Design review of the part shown in the three views and the two pictorial views. Dimensions are in mm from the part's minimum x, y and z. Round coordinates to 2 decimals unless told otherwise and drop trailing zeros. Loops run counter-clockwise (first coordinate to the right, second up) from the corner with the lowest first, then second, coordinate; pieces in that order, holes last.
1. Consider section A-A on x = 22.5. State the section outline as (y, z) points, then the cut area to 3 significant figures.
2. Clearance check with a flat-ended pin moving along its axis: pin 1 Ø2.5 at (x, z) = (22.5, 25) entering from +Y. State where the tip first meets the part, or that it passes through.
3. Consider section D-D on x = 7.5. State the section outline as (y, z) points.
4. To check wall thickness, follow line 1 along X through (y, z) = (0.8, 36.5); line 2 along Z through (x, y) = (37.5, 1.95); line 3 along Z through (x, y) = (6, 0.6). State the ranges of each line that lie inside material, in increasing order.
5. Consider section B-B on y = 1.1. State the section outline as (x, z) points.
6. Consider section C-C on z = 25. State the section outline as (x, y) points.
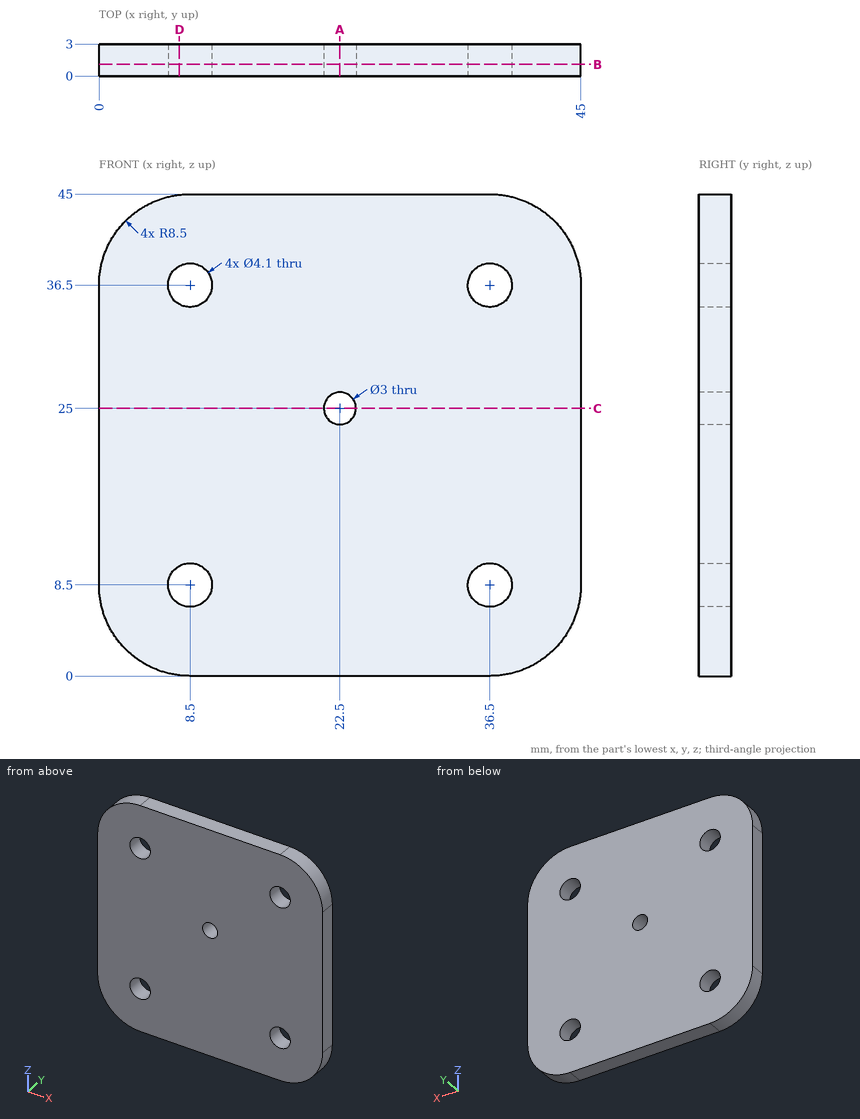
Resolved:
1. outline: (0, 0) - (3, 0) - (3, 23.5) - (0, 23.5) - close; (0, 26.5) - (3, 26.5) - (3, 45) - (0, 45) - close
1. area: 126 mm2
2. pin 1: passes through
3. outline: (0, 0.06) - (3, 0.06) - (3, 6.71) - (0, 6.71) - close; (0, 10.29) - (3, 10.29) - (3, 34.71) - (0, 34.71) - close; (0, 38.29) - (3, 38.29) - (3, 44.94) - (0, 44.94) - close
4. line 1: x = 0 to 6.45, 10.55 to 34.45, 38.55 to 45
4. line 2: z = 0.06 to 6.71, 10.29 to 34.71, 38.29 to 44.94
4. line 3: z = 0.38 to 44.62
5. outline: (0, 8.5) arc R8.5 ccw to (8.5, 0) - (36.5, 0) arc R8.5 ccw to (45, 8.5) - (45, 36.5) arc R8.5 ccw to (36.5, 45) - (8.5, 45) arc R8.5 ccw to (0, 36.5) - close; hole circle Ø4.1 at (8.5, 8.5); hole circle Ø4.1 at (8.5, 36.5); hole circle Ø3 at (22.5, 25); hole circle Ø4.1 at (36.5, 8.5); hole circle Ø4.1 at (36.5, 36.5)
6. outline: (0, 0) - (21, 0) - (21, 3) - (0, 3) - close; (24, 0) - (45, 0) - (45, 3) - (24, 3) - close
